from build123d import *

# Parameters (mm, degrees)
BOSS_EXTRUDE1_DEPTH = 1.5875
SKETCH4_R           = 2.032
CUT_EXTRUDE1_DEPTH  = 1.5875


with BuildPart() as part:
    # Sketch3 → Boss-Extrude1 (new body)
    with BuildSketch(Plane(origin=(0, 0, 0), x_dir=(1, 0, 0), z_dir=(0, 1, 0))):
        Polygon((0, 0), (101.6, 0), (101.6, -25.4), (76.2, -25.4), (76.2, -76.2), (25.4, -76.2), (25.4, -25.4), (0, -25.4), align=None)
    extrude(amount=BOSS_EXTRUDE1_DEPTH)

    # Sketch4 → Cut-Extrude1 (cut)
    with BuildSketch(Plane(origin=(0, 1.5875, 0), x_dir=(1, 0, 0), z_dir=(0, 1, 0))):
        with Locations((6.35, -6.35)):
            Circle(SKETCH4_R)
        with Locations((19.05, -6.35)):
            Circle(SKETCH4_R)
        with Locations((82.55, -6.35)):
            Circle(SKETCH4_R)
        with Locations((95.25, -6.35)):
            Circle(SKETCH4_R)
        with Locations((107.95, -6.35)):
            Circle(SKETCH4_R)
        with Locations((120.65, -6.35)):
            Circle(SKETCH4_R)
        with Locations((133.35, -6.35)):
            Circle(SKETCH4_R)
        with Locations((146.05, -6.35)):
            Circle(SKETCH4_R)
        with Locations((19.05, -19.05)):
            Circle(SKETCH4_R)
        with Locations((82.55, -19.05)):
            Circle(SKETCH4_R)
        with Locations((95.25, -19.05)):
            Circle(SKETCH4_R)
        with Locations((107.95, -19.05)):
            Circle(SKETCH4_R)
        with Locations((120.65, -19.05)):
            Circle(SKETCH4_R)
        with Locations((133.35, -19.05)):
            Circle(SKETCH4_R)
        with Locations((146.05, -19.05)):
            Circle(SKETCH4_R)
        with Locations((19.05, -31.75)):
            Circle(SKETCH4_R)
        with Locations((31.75, -31.75)):
            Circle(SKETCH4_R)
        with Locations((69.85, -31.75)):
            Circle(SKETCH4_R)
        with Locations((82.55, -31.75)):
            Circle(SKETCH4_R)
        with Locations((95.25, -31.75)):
            Circle(SKETCH4_R)
        with Locations((107.95, -31.75)):
            Circle(SKETCH4_R)
        with Locations((120.65, -31.75)):
            Circle(SKETCH4_R)
        with Locations((133.35, -31.75)):
            Circle(SKETCH4_R)
        with Locations((146.05, -31.75)):
            Circle(SKETCH4_R)
        with Locations((19.05, -44.45)):
            Circle(SKETCH4_R)
        with Locations((31.75, -44.45)):
            Circle(SKETCH4_R)
        with Locations((69.85, -44.45)):
            Circle(SKETCH4_R)
        with Locations((82.55, -44.45)):
            Circle(SKETCH4_R)
        with Locations((95.25, -44.45)):
            Circle(SKETCH4_R)
        with Locations((107.95, -44.45)):
            Circle(SKETCH4_R)
        with Locations((120.65, -44.45)):
            Circle(SKETCH4_R)
        with Locations((133.35, -44.45)):
            Circle(SKETCH4_R)
        with Locations((146.05, -44.45)):
            Circle(SKETCH4_R)
        with Locations((19.05, -57.15)):
            Circle(SKETCH4_R)
        with Locations((31.75, -57.15)):
            Circle(SKETCH4_R)
        with Locations((69.85, -57.15)):
            Circle(SKETCH4_R)
        with Locations((82.55, -57.15)):
            Circle(SKETCH4_R)
        with Locations((95.25, -57.15)):
            Circle(SKETCH4_R)
        with Locations((107.95, -57.15)):
            Circle(SKETCH4_R)
        with Locations((120.65, -57.15)):
            Circle(SKETCH4_R)
        with Locations((133.35, -57.15)):
            Circle(SKETCH4_R)
        with Locations((146.05, -57.15)):
            Circle(SKETCH4_R)
        with Locations((19.05, -69.85)):
            Circle(SKETCH4_R)
        with Locations((31.75, -69.85)):
            Circle(SKETCH4_R)
        with Locations((44.45, -69.85)):
            Circle(SKETCH4_R)
        with Locations((57.15, -69.85)):
            Circle(SKETCH4_R)
        with Locations((69.85, -69.85)):
            Circle(SKETCH4_R)
        with Locations((82.55, -69.85)):
            Circle(SKETCH4_R)
        with Locations((95.25, -69.85)):
            Circle(SKETCH4_R)
        with Locations((107.95, -69.85)):
            Circle(SKETCH4_R)
        with Locations((120.65, -69.85)):
            Circle(SKETCH4_R)
        with Locations((133.35, -69.85)):
            Circle(SKETCH4_R)
        with Locations((146.05, -69.85)):
            Circle(SKETCH4_R)
        with Locations((6.35, -19.05)):
            Circle(SKETCH4_R)
        with Locations((6.35, -31.75)):
            Circle(SKETCH4_R)
        with Locations((6.35, -44.45)):
            Circle(SKETCH4_R)
        with Locations((6.35, -57.15)):
            Circle(SKETCH4_R)
        with Locations((6.35, -69.85)):
            Circle(SKETCH4_R)
    extrude(amount=-CUT_EXTRUDE1_DEPTH, mode=Mode.SUBTRACT)


solid = part.part
The model under review builds one solid part; all positions refer to its coordinate system, in mm. Round coordinates to 2 decimals unless told otherwise and drop trailing zeros. Loops run counter-clockwise (first coordinate to the right, second up) from the corner with the lowest first, then second, coordinate; pieces in that order, holes last. Notation, with made-up numbers: (40.5, 80) -> (45.5, 80) arc R14 ccw to (45.5, 90) -> close; hole circle Ø2 at (49, 8.5). An arc over 180 degrees is marked (long way). Answer as CSV lines item,"result".
1) Add section A-A on x = 6.35. Write out the cut boundary in (y, z), plus the area to 3 significant figures.
Geometry results:
outline,"(0, 0) -> (1.59, 0) -> (1.59, 4.32) -> (0, 4.32) -> close; (0, 8.38) -> (1.59, 8.38) -> (1.59, 17.02) -> (0, 17.02) -> close; (0, 21.08) -> (1.59, 21.08) -> (1.59, 25.4) -> (0, 25.4) -> close"
area,"27.4 mm²"
2) For P1, Ø0.5, axis at x = 11, y = 0.5, coming from the +Z side; P2, Ø0.8, axis at y = 0.5, z = 52, coming from the +X side, all flat-tipped, find the tip position at first contact; note any pin that passes through.
Geometry results:
P1,"stops at z = 25.4"
P2,"stops at x = 76.2"
3) Add section B-B on x = 44.45. Write out the cut boundary in (y, z), plus the area to 3 significant figures.
Geometry results:
outline,"(0, 0) -> (1.59, 0) -> (1.59, 67.82) -> (0, 67.82) -> close; (0, 71.88) -> (1.59, 71.88) -> (1.59, 76.2) -> (0, 76.2) -> close"
area,"115 mm²"
4) To check wall thickness, follow line 1 along Z through (x, y) = (31.75, 0.95); line 2 along Z through (x, y) = (6.5, 1.35); line 3 along X through (y, z) = (1.1, 19.05). State the ranges of each line that lie inside material, in increasing order. Write a range as from..to.
Geometry results:
line 1,"z = 0..29.72, 33.78..42.42, 46.48..55.12, 59.18..67.82, 71.88..76.2"
line 2,"z = 0..4.32, 8.38..17.02, 21.08..25.4"
line 3,"x = 0..4.32, 8.38..17.02, 21.08..80.52, 84.58..93.22, 97.28..101.6"
5) Add section C-C on y = 0.25. State how many separate pieces and enclosed holes the cut face has, plus the area to 3 significant figures.
Geometry results:
separate pieces,"1"
enclosed holes,"18"
area,"4,930 mm²"
6) Draft analysis for pull direction X (two halves, no side actions). For faces 1 (the face through (32.69, 0.8, 58.95)), 2 (the face through (32.842, 0.805, 30.037)), 3 (the face through (52, 1.588, 29)), state which applies: pulls with the +X half, pulls with the -X half, needs draft (parallel to the pull), parting line crosses it, or undercut.
Geometry results:
face 1,"undercut"
face 2,"undercut"
face 3,"needs draft"
7) Add section D-D on z = 63.5. Write out the cut boundary in (x, y), plus the area to 3 significant figures.
Geometry results:
outline,"(25.4, 0) -> (76.2, 0) -> (76.2, 1.59) -> (25.4, 1.59) -> close"
area,"80.6 mm²"
